from build123d import *

# Parameters (mm, degrees)
F0_R          = 14.2875
F0_R_2        = 12.5
F1_DEPTH      = 101.6
F1_DEPTH_BACK = 101.6
F0_R_3        = 3.96875
F2_DEPTH      = 203.2
F2_DEPTH_BACK = 127
F3_DEPTH      = 25.4


with BuildPart() as f1:
    # F0 (on Right) → F1 (new body, two sides)
    with BuildSketch(Plane.YZ) as f1_sk:
        Circle(F0_R)
        Circle(F0_R_2, mode=Mode.SUBTRACT)
    extrude(amount=F1_DEPTH)
    extrude(f1_sk.sketch, amount=-F1_DEPTH_BACK)

    # F0 (on Right) → F2 (join, two sides)
    with BuildSketch(Plane.YZ) as f2_sk:
        Circle(F0_R_2)
        Circle(F0_R_3, mode=Mode.SUBTRACT)
    extrude(amount=F2_DEPTH)
    extrude(f2_sk.sketch, amount=-F2_DEPTH_BACK)

    # F0 (on Right) → F3 (join)
    with BuildSketch(Plane.YZ):
        Circle(F0_R_3)
    extrude(amount=F3_DEPTH)


solid = f1.part
Read the model definition and answer for the solid it produces. Units are mm, in the model's axes. A direction names the side the tool comes from. Give positions to 0.01 mm unless a question says otherwise; leave off trailing zeros. Loops run counter-clockwise (first coordinate to the right, second up) from the corner with the lowest first, then second, coordinate; pieces in that order, holes last. Notation, with made-up numbers: (-39, 3.5) -> (14, 3.5) arc R20 ccw to (14, 10.5) -> close; hole circle Ø6 at (64.5, 16). An arc over 180 degrees is marked (long way). Use a Markdown table: item, result.
Q1. Each of these flat-tipped pins is pushed along its axis until it touches: pin 1 (1 mm diameter, centred on x = -76.5, y = -6, fed in from +Z); pin 2 (10 mm diameter, centred on x = 159, y = -3, fed in from +Z); pin 3 (12 mm diameter, centred on x = 85, y = -3, fed in from +Z); pin 4 (1.5 mm diameter, centred on x = 103, z = 1, fed in from -Y). Where does it stop, or does it pass through?
Solved:
| item | result |
|---|---|
| pin 1 | stops at z = 13.19 |
| pin 2 | stops at z = 12.5 |
| pin 3 | stops at z = 14.29 |
| pin 4 | stops at y = -12.5 |
Q2. Section A-A, the plane z = 0 is taken. Determine the outline of the cut face in (x, y).
Solved:
| item | result |
|---|---|
| outline | (-127, -12.5) -> (-101.6, -12.5) -> (-101.6, -14.29) -> (101.6, -14.29) -> (101.6, -12.5) -> (203.2, -12.5) -> (203.2, -3.97) -> (25.4, -3.97) -> (25.4, 3.97) -> (203.2, 3.97) -> (203.2, 12.5) -> (101.6, 12.5) -> (101.6, 14.29) -> (-101.6, 14.29) -> (-101.6, 12.5) -> (-127, 12.5) -> (-127, 3.97) -> (0, 3.97) -> (0, -3.97) -> (-127, -3.97) -> close |
Q3. Section D-D, the plane x = 63.5 is taken. Determine the outline of the cut face in (y, z) (1 decimal).
Solved:
| item | result |
|---|---|
| outline | circle Ø28.6 at (0, 0); hole circle Ø7.9 at (0, 0) |
Q4. Find the intervals of material crossed by line 1 along Z through (x, y) = (80, 0); line 2 along Z through (x, y) = (117, 0); line 3 along X through (y, z) = (12.25, -6), in increasing order.
Solved:
| item | result |
|---|---|
| line 1 | z = -14.29 to -3.97, 3.97 to 14.29 |
| line 2 | z = -12.5 to -3.97, 3.97 to 12.5 |
| line 3 | x = -101.6 to 101.6 |
Q5. Section C-C, the plane x = 144.5 is taken. Determine the outline of the cut face in (y, z), then the cut area to 3 significant figures.
Solved:
| item | result |
|---|---|
| outline | circle Ø25 at (0, 0); hole circle Ø7.94 at (0, 0) |
| area | 441 mm^2 |
Q6. A tool of negligible diameter and unlimited length cuts with its end or side. For faces 4 (the face through (113.055, -0.86, -3.874)), 5 (the face through (-62.611, -0.86, -3.874)), 6 (the face through (1.422, -14.274, 0.628)), from which of +Z, -Z, +X, -X, +Y, -Y can it reach the whole face along a straight path? Write none if from no direction.
Solved:
| item | result |
|---|---|
| face 4 | +X |
| face 5 | -X |
| face 6 | +X, -X |
Q7. Determine the mould class of faces 1 (the face through (151.689, 11.923, 3.755)), 2 (the face through (-101.6, 0, -13)), 3 (the face through (25.4, 0, 0)) for opening direction Y: pulls with the +Y half, pulls with the -Y half, needs draft (parallel to the pull), parting line crosses it, or undercut.
Solved:
| item | result |
|---|---|
| face 1 | parting line crosses it |
| face 2 | needs draft |
| face 3 | undercut |
